Autodesk Inventor part; units mm, degrees
ref_plane "YZ Plane" through (0, 0, 0) normal (1, 0, 0) x (0, 1, 0)
ref_plane "XZ Plane" through (0, 0, 0) normal (0, 1, 0) x (-1, 0, 0)
ref_plane "XY Plane" through (0, 0, 0) normal (0, 0, 1) x (1, 0, 0)
sketch "Sketch1" plane through (0, 0, 0) normal (1, 0, 0) x (0, 1, 0)
  circle A0 centre (0, 0) radius 4.75
  line L0 (10, 45) -> (-10, 45)
  line L1 (10, 38) -> (-10, 38)
  line L2 (10, 45) -> (10, 38)
  line L3 (-10, 38) -> (-10, 45)
  line L4 (-4.75, 0) -> (-8.4137, 0)
  line L5 (-14, 0) -> (14, 0)
  line L6 (10, -55) -> (-10, -55)
  line L7 (-10, -55) -> (-10, -48)
  line L8 (-10, -48) -> (10, -48)
  line L9 (10, -48) -> (10, -55)
  line L10 (10, 38) -> (10, -48)
  line L11 (-10, -48) -> (-10, 38)
  point P0 (0, 45)
  point P1 (0, -55)
  dimension "d0" = 9.5
  dimension "d1" = 20
  dimension "d2" = 0
  dimension "d3" = 7
  dimension "d4" = 45
  dimension "d8" = 20
  dimension "d9" = 7
  dimension "d10" = 0
  dimension "d11" = 55
extrude "Extrusion1" add sketch "Sketch1" along normal blind 10 contours L5 L10 L8 L11 L4 A0 | A0 L4 L5 L11 L1 L10 | L1 L3 L0 L2 | L9 L6 L7 L8
sketch "Sketch2" plane through (0, -10, -55) normal (0, 0, -1) x (-1, 0, 0)
  circle A0 centre (-5, 10) radius 2.475
  point P0 (0, 10)
  dimension "d12" = 4.95
extrude "Extrusion2" add sketch "Sketch2" along normal blind 4.9
chamfer "Chamfer1" distance 0.5 angle 45 1 edges at (7.475, 0, -59.9)
sketch "Sketch3" plane through (0, -10, -55) normal (0, 0, -1) x (-1, 0, 0)
  circle A0 centre (-5, 10) radius 2.475
  circle A1 centre (-5, 10) radius 7
  circle A2 centre (-5, 10) radius 17.4724
  point P0 (0, 10)
  dimension "d18" = 14
extrude "Extrusion3" cut sketch "Sketch3" against normal through all contours A2
properties part number "temp_nozzle_v2"
Read the model definition and answer for the solid it produces. Units are mm, in the model's axes. A direction names the side the tool comes from. Give positions to 0.01 mm unless a question says otherwise; leave off trailing zeros. Write each loop counter-clockwise with the first axis right and the second up, starting at its lowest first coordinate (ties: lowest second). Pieces come first, ordered by that corner, then holes. Notation, with made-up numbers: (86.5, -29) -> (130.5, -29) arc R20 cw to (130.5, -6) -> close; hole circle Ø6 at (-6, 56). An arc over 180 degrees is marked (long way). Answer in a Markdown table with one row per item.
1) Section C-C on z = -33.5 is taken. Give the vertices of the cut face in (x, y).
Results list:
| item | result |
|---|---|
| outline | (0, -4.9) arc R7 ccw to (10, -4.9) -> (10, 4.9) arc R7 ccw to (0, 4.9) -> close |
2) A tool of negligible diameter and unlimited length cuts with its end or side. For faces 5 (the flat face through (0, 3, -4)), 6 (the cylindrical face through (2.64, -0.74, -57.17)), from which of +Z, -Z, +X, -X, +Y, -Y can it reach the whole face along a straight path? Write none if from no direction.
Results list:
| item | result |
|---|---|
| face 5 | +Z, -Z, -X, +Y, -Y |
| face 6 | -Z |
3) Section D-D on x = 1 is taken. Give the vertices of the cut face in (y, z).
Results list:
| item | result |
|---|---|
| outline | (-5.74, -55) -> (5.74, -55) -> (5.74, 45) -> (-5.74, 45) -> close; hole circle Ø9.5 at (0, 0) |
4) Determine the mould class of faces 1 (the cylindrical face through (4.93, 2.192, 4.214)), 2 (the cylindrical face through (5, 7, -6)), 3 (the flat face through (5, 0, 45)), 4 (the flat face through (5, 0, -59.9)) for opening direction Z: released by +Z, released by -Z, zero draft, split by the parting line, or undercut.
Results list:
| item | result |
|---|---|
| face 1 | undercut |
| face 2 | zero draft |
| face 3 | released by +Z |
| face 4 | released by -Z |
5) Straight lines are drawn through the part: line 1 (Z direction, x = 5.5, y = 0); line 2 (Z direction, x = 4.25, y = -6.5); line 3 (Y direction, x = 3, z = 0). For each, find the intervals that lie inside material, in ascending order. Write a range as [from, to].
Results list:
| item | result |
|---|---|
| line 1 | [-59.9, -4.75], [4.75, 45] |
| line 2 | [-55, 45] |
| line 3 | [-6.71, -4.75], [4.75, 6.71] |
6) Section B-B on x = 5 is taken. Give the vertices of the cut face in (y, z) (3 decimals), plus the area to 3 significant figures.
Results list:
| item | result |
|---|---|
| outline | (-7, -55) -> (-2.475, -55) -> (-2.475, -59.4) -> (-1.975, -59.9) -> (1.975, -59.9) -> (2.475, -59.4) -> (2.475, -55) -> (7, -55) -> (7, 45) -> (-7, 45) -> close; hole circle Ø9.5 at (0, 0) |
| area | 1,350 mm^2 |
7) Section A-A on y = 0 is taken. Give the vertices of the cut face in (x, z) (3 decimals), plus the area to 3 significant figures.
Results list:
| item | result |
|---|---|
| outline | (0, -55) -> (2.525, -55) -> (2.525, -59.4) -> (3.025, -59.9) -> (6.975, -59.9) -> (7.475, -59.4) -> (7.475, -55) -> (10, -55) -> (10, -4.75) -> (0, -4.75) -> close; (0, 4.75) -> (10, 4.75) -> (10, 45) -> (0, 45) -> close |
| area | 929 mm^2 |
8) This flat-tipped pin is pushed along its axis until it touches: pin 1 Ø1 at (x, z) = (9, -31.5) entering from +Y. Where does it stop, or does it pass through?
Results list:
| item | result |
|---|---|
| pin 1 | y = 6.06 |
